Input: part model. Units: mm. Frame: model coordinates. Coordinates: 2 decimals unless noted, no trailing zeros. Order: outer loops, then holes, each group sorted by start corner. A loop starts at its lowest first (then second) coordinate and runs counter-clockwise, first axis right, second up.
from build123d import *


with BuildPart() as part:
    # Sketch1 → Revolve1 (revolve)
    with BuildSketch(Plane(origin=(0, 0, 0), x_dir=(1, 0, 0), z_dir=(0, 1, 0)), mode=Mode.PRIVATE) as revolve1_sk:
        Polygon((18.415, 129.963013839), (18.415, 128.496544155), (44.3992, 143.49852902), (41.8592, 143.49852902), align=None)
        Polygon((44.3992, 96.750377662), (44.3992, 114.3), (44.3992, 143.49852902), (18.415, 128.496544155), (18.415, 120.876544155), (32.07390948, 69.9008), (39.664895038, 69.9008), (40.777169393, 76.208821327), align=None)
    revolve(revolve1_sk.sketch.rotate(Axis((0, 0, -147.178415471), (0, 0, 1)), 180), axis=Axis((0, 0, -147.178415471), (0, 0, 1)))


solid = part.part
Item 1: Cut plane B-B on z = -116. Return loops of the section in (x, y), then the cut area to 3 significant figures.
Response values:
outline: circle Ø88.8 at (0, 0); hole circle Ø39.44 at (0, 0)
area: 4,970 mm2
Item 2: Ray query, probe 1 along Y at (x, z) = (0, -124) (3 decimals); probe 2 along X at (y, z) = (-11.5, -103.5); probe 3 along X at (y, z) = (15.5, -132). Return the intervals inside material, ascending.
Response values:
probe 1: y = -44.399 to -18.415, 18.415 to 44.399
probe 2: x = -42.88 to -20, 20 to 42.88
probe 3: x = -41.61 to -15.53, 15.53 to 41.61
Item 3: Cut plane A-A on z = -126. Return loops of the section in (x, y) (3 decimals), then the cut area to 3 significant figures.
Response values:
outline: circle Ø88.798 at (0, 0); hole circle Ø36.83 at (0, 0)
area: 5,130 mm2
Item 4: Draft query along Y for faces 1 (the face through (-18.06, 7.49, -130.62)), 2 (the face through (-3.1, 32.1, -69.901)), 3 (the face through (-20.49, 39.39, -120.45)). Return one class per face: pulls with the +Y half, pulls with the -Y half, needs draft (parallel to the pull), parting line crosses it, or undercut.
Response values:
face 1: undercut
face 2: needs draft
face 3: parting line crosses it
Item 5: Pin query (flat end, axial travel): pin 1 Ø22 at (x, y) = (0, 0) entering from -Z (3 decimals); pin 2 Ø10 at (x, y) = (19, -29) entering from -Z; pin 3 Ø2 at (y, z) = (-34.5, -106.5) entering from +X; pin 4 Ø12 at (x, z) = (22.5, -115) entering from -Y. Return the tip coordinate at first contact, or that it passes through.
Response values:
pin 1: passes through
pin 2: stops at z = -142.23
pin 3: stops at x = 29.14
pin 4: stops at y = -41.22
